Input: part model. Units: mm. Frame: model coordinates. A direction names the side the tool comes from. Round coordinates to 2 decimals unless told otherwise and drop trailing zeros. Loops run counter-clockwise (first coordinate to the right, second up) from the corner with the lowest first, then second, coordinate; pieces in that order, holes last.
(1) Line query: line 1 (Y direction, x = 9, z = -1.25); line 2 (X direction, y = 36, z = -0.25); line 3 (Z direction, x = 2.25, y = 99.5). Output: solid intervals per line, ascending.
(2) Cut plane A-A, the plane z = 0. Output: boundary loops of the cut face in (x, y).
(3) First-contact query: pin 1 Ø10 at (x, z) = (-7.5, 3.5) entering from -Y; pin 2 Ø5 at (y, z) = (15, -7.5) entering from -X; pin 3 Ø6 at (x, y) = (7.5, 99.5) entering from -Z; pin 4 Ø1 at (x, z) = (-3.5, 6) entering from +Y. Flat tips, straight axial feed; report the tip coordinate or a pass-through.
(4) Access query for faces 1 (the face through (0, 115, 0)), 2 (the face through (5, 0, 2)). Directions: +Z, -Z, +X, -X, +Y, -Y. A direction counts if a zero-diameter tool reaches every point of the face in a straight line with its end or side. Return the directions, or none.
(5) Cut plane B-B, the plane x = 0. Output: boundary loops of the cut face in (y, z), and give its area (3 significant figures).
(6) Cut plane D-D, the plane z = -8. Output: boundary loops of the cut face in (x, y), and give its area (3 significant figures).
(7) Cut plane C-C, the plane y = 58.5. Output: boundary loops of the cut face in (x, z), and give its area (3 significant figures).
(8) Draft query along Y for faces 3 (the face through (-4.88, 112.46, -1.08)), 4 (the face through (5, 110, 2)), 5 (the face through (0, -5, 0)). Return one class per face: released by +Y, released by -Y, zero draft, split by the parting line, or undercut.
from build123d import *

# Parameters (mm, degrees)
SKETCH2_R           = 10
SKETCH2_R_2         = 5
BOSS_EXTRUDE1_DEPTH = 110
SKETCH2_2_R         = 5
BOSS_EXTRUDE2_DEPTH = 115
BOSS_EXTRUDE3_START = -5
SKETCH2_3_R         = 5
BOSS_EXTRUDE3_DEPTH = 5


with BuildPart() as part:
    # Sketch2 → Boss-Extrude1 (new body)
    with BuildSketch(Plane(origin=(0, 0, 0), x_dir=(1, 0, 0), z_dir=(0, 1, 0))):
        with Locations(Location((0, 0, 0), (0, 0, 270))):
            Circle(SKETCH2_R)
        with Locations(Location((0, 0, 0), (0, 0, 270))):
            Circle(SKETCH2_R_2, mode=Mode.SUBTRACT)
    extrude(amount=BOSS_EXTRUDE1_DEPTH)

    # Sketch2_2 → Boss-Extrude2 (add)
    with BuildSketch(Plane(origin=(0, 0, 0), x_dir=(1, 0, 0), z_dir=(0, 1, 0))):
        with Locations(Location((0, 0, 0), (0, 0, 270))):
            Circle(SKETCH2_2_R)
    extrude(amount=BOSS_EXTRUDE2_DEPTH)

    # Sketch2_3 → Boss-Extrude3 (add)
    with BuildSketch(Plane(origin=(0, 0, 0), x_dir=(1, 0, 0), z_dir=(0, 1, 0)).offset(BOSS_EXTRUDE3_START)):
        with Locations(Location((0, 0, 0), (0, 0, 270))):
            Circle(SKETCH2_3_R)
    extrude(amount=BOSS_EXTRUDE3_DEPTH)


solid = part.part
Reported:
1. line 1: y = 0 to 110
1. line 2: x = -10 to 10
1. line 3: z = -9.74 to 9.74
2. outline: (-10, 0) - (-5, 0) - (-5, -5) - (5, -5) - (5, 0) - (10, 0) - (10, 110) - (5, 110) - (5, 115) - (-5, 115) - (-5, 110) - (-10, 110) - close
3. pin 1: stops at y = -5
3. pin 2: stops at x = -8.66
3. pin 3: stops at z = -8.93
3. pin 4: stops at y = 110
4. face 1: +Z, -Z, +X, -X, +Y
4. face 2: -Y
5. outline: (-5, -5) - (0, -5) - (0, -10) - (110, -10) - (110, -5) - (115, -5) - (115, 5) - (110, 5) - (110, 10) - (0, 10) - (0, 5) - (-5, 5) - close
5. area: 2,300 mm2
6. outline: (-6, 0) - (6, 0) - (6, 110) - (-6, 110) - close
6. area: 1,320 mm2
7. outline: circle Ø20 at (0, 0)
7. area: 314 mm2
8. face 3: zero draft
8. face 4: released by +Y
8. face 5: released by -Y
